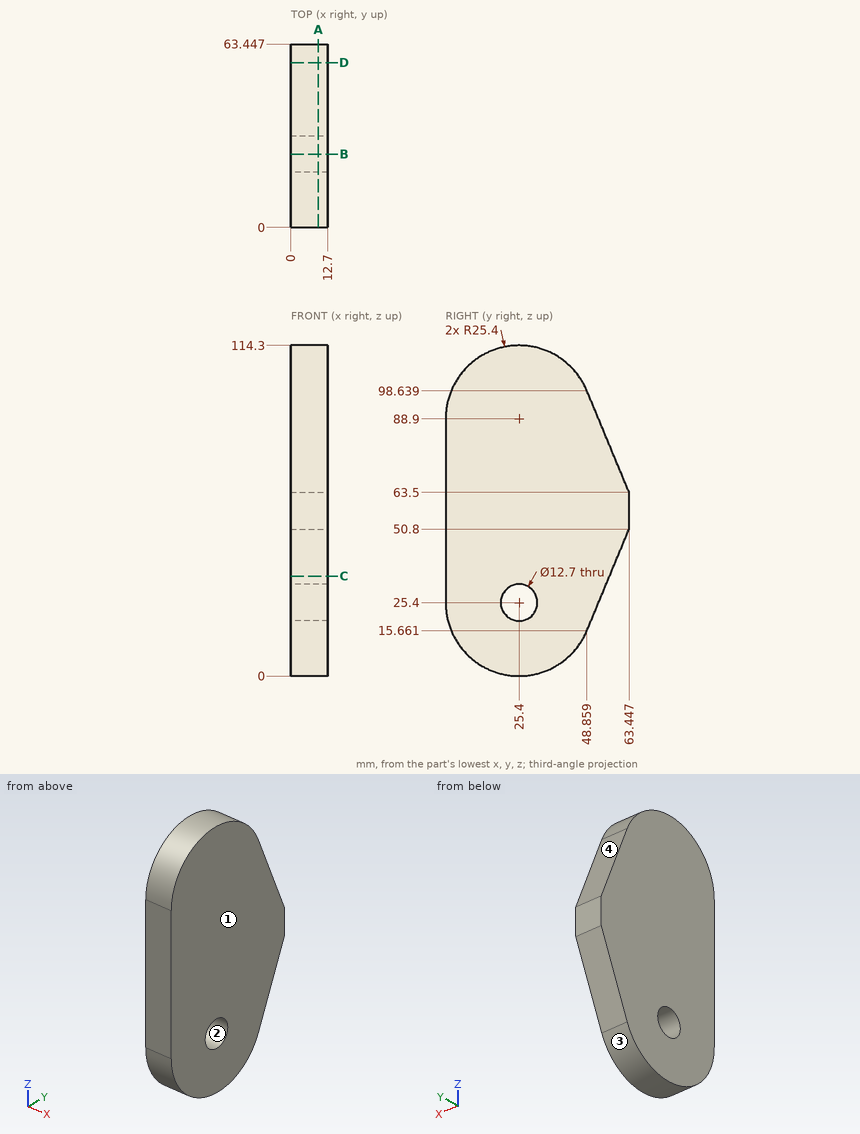
Study the drawing (mm; zero at the part's minimum x, y, z) and answer. Round coordinates to 2 decimals unless told otherwise and drop trailing zeros. Write each loop counter-clockwise with the first axis right and the second up, starting at its lowest first coordinate (ties: lowest second). Pieces come first, ordered by that corner, then holes.
1) The mould has two halves that part along Y. Classify the marked faces 1, 2, 3 and 4: pulls with the +Y half, pulls with the -Y half, needs draft (parallel to the pull), parting line crosses it, or undercut.
2) A cutting plane is placed at A-A (x = 9.5). Give the vertices of the cut face in (y, z).
3) A cutting plane is placed at B-B (y = 25.4). Give the vertices of the cut face in (x, z).
4) Given pin 1 Ø1.5 at (x, z) = (2.5, 82.5) entering from +Y; pin 2 Ø5 at (x, z) = (1.5, 25) entering from +Y; pin 3 Ø3 at (x, y) = (4, 15.5) entering from +Z, each flat-ended and moving along its own axis, determine where each tip first touches the part or whether it passes through.
5) A cutting plane is placed at D-D (y = 57). Give the vertices of the cut face in (x, z), plus the area to 3 significant figures.
6) Straight lines are drawn through the part: line 1 (Z direction, x = 8.25, y = 25.4); line 2 (Y direction, x = 6, z = 25.4); line 3 (Y direction, x = 2.75, z = 29). For each, find the intervals that lie inside material, in ascending order.
7) A cutting plane is placed at C-C (z = 34.5). Give the vertices of the cut face in (x, y), plus the area to 3 significant figures.
Completed:
1. face 1: needs draft
1. face 2: undercut
1. face 3: parting line crosses it
1. face 4: pulls with the +Y half
2. outline: (0, 25.4) arc R25.4 ccw to (48.86, 15.66) - (63.45, 50.8) - (63.45, 63.5) - (48.86, 98.64) arc R25.4 ccw to (0, 88.9) - close; hole circle Ø12.7 at (25.4, 25.4)
3. outline: (0, 0) - (12.7, 0) - (12.7, 19.05) - (0, 19.05) - close; (0, 31.75) - (12.7, 31.75) - (12.7, 114.3) - (0, 114.3) - close
4. pin 1: stops at y = 55.87
4. pin 2: stops at y = 53.77
4. pin 3: stops at z = 112.87
5. outline: (0, 35.27) - (12.7, 35.27) - (12.7, 79.03) - (0, 79.03) - close
5. area: 556 mm2
6. line 1: z = 0 to 19.05, 31.75 to 114.3
6. line 2: y = 0 to 19.05, 31.75 to 52.9
6. line 3: y = 0 to 20.17, 30.63 to 54.4
7. outline: (0, 0) - (12.7, 0) - (12.7, 56.68) - (0, 56.68) - close
7. area: 720 mm2
